Here's how the part is built. I have some questions about the finished solid (model axes, mm). Face numbers are marked on the shaded views. A direction names the side the tool comes from. Round coordinates to 2 decimals unless told otherwise and drop trailing zeros. Loops run counter-clockwise (first coordinate to the right, second up) from the corner with the lowest first, then second, coordinate; pieces in that order, holes last. Notation, with made-up numbers: (-12.5, -20) -> (15.5, -20) arc R22 ccw to (15.5, 14) -> close; hole circle Ø11 at (17.5, 25.5). An arc over 180 degrees is marked (long way). Use CSV: the item, a comma, the result in double quotes. Start each with the question number.
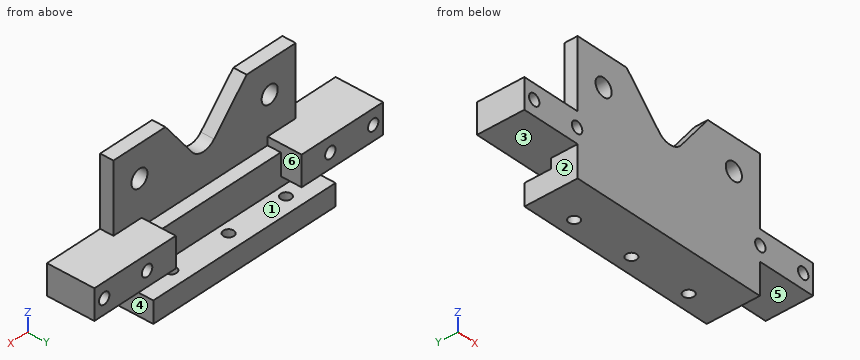
Autodesk Inventor part; units mm, degrees
ref_plane "YZ Plane" through (0, 0, 0) normal (1, 0, 0) x (0, 1, 0)
ref_plane "XZ Plane" through (0, 0, 0) normal (0, 1, 0) x (-1, 0, 0)
ref_plane "XY Plane" through (0, 0, 0) normal (0, 0, 1) x (1, 0, 0)
ref_plane "Work Plane1" through (-0.2015, 0, 0) normal (0, 0, 1) x (1, 0, 0)
sketch "Sketch1" plane through (-0.2015, 0, 0) normal (0, 0, 1) x (1, 0, 0)
  circle A0 centre (19.4801, 3.175) radius 1.0541
  circle A1 centre (44.8801, 3.175) radius 1.0541
  circle A2 centre (57.5801, 3.175) radius 1.0541 construction
  circle A3 centre (6.7801, 3.175) radius 1.0541 construction
  circle A4 centre (32.1801, 3.175) radius 1.0541
  line L0 (0.2015, 0) -> (64.1587, 0) construction
  line L1 (64.1587, 0) -> (64.1587, 6.35) construction
  line L2 (0.2015, 6.35) -> (64.1587, 6.35) construction
  line L3 (0.2015, 0) -> (0.2015, 6.35) construction
  line L4 (52.3672, 6.35) -> (11.9931, 6.35)
  line L5 (11.9931, 6.35) -> (11.9931, 0)
  line L6 (11.9931, 0) -> (52.3672, 0)
  line L7 (52.3672, 0) -> (52.3672, 6.35)
  line L8 (44.8801, 3.175) -> (52.3672, 3.175) construction
  line L9 (19.4801, 3.175) -> (11.9931, 3.175) construction
extrude "Extrusion1" add sketch "Sketch1" along normal blind 4.318
sketch "Sketch2" plane through (11.7916, 0, 0) normal (0, -1, 0) x (1, 0, 0)
  line L0 (0, 0) -> (40.3741, 0)
  line L1 (40.3741, 0) -> (40.3741, 4.318)
  line L2 (0, 4.318) -> (40.3741, 4.318)
  line L3 (0, 0) -> (0, 4.318)
  point P0 (-11.7916, 0)
extrude "Extrusion2" add sketch "Sketch2" along normal blind 4.318
sketch "Sketch3" plane through (-0.2015, 0, 4.318) normal (0, 0, 1) x (1, 0, 0)
  line L0 (52.3672, 6.35) -> (52.3672, -4.318)
  line L1 (52.3672, 1.016) -> (11.9931, 1.016)
  line L2 (11.9931, 6.35) -> (11.9931, -4.318)
  line L3 (52.3672, -4.318) -> (11.9931, -4.318)
  line L4 (52.3672, 1.016) -> (11.9931, 1.016)
  line L5 (11.9931, 1.016) -> (11.9931, -4.318)
  line L6 (11.9931, -4.318) -> (52.3672, -4.318)
  line L7 (52.3672, -4.318) -> (52.3672, 1.016)
  point P0 (0.2015, 0)
extrude "Extrusion3" add sketch "Sketch3" along normal blind 21.7805
sketch "Sketch4" plane through (11.7916, -4.318, 0) normal (0, -1, 0) x (1, 0, 0)
  line L0 (0, 0) -> (40.3741, 0) construction
  line L1 (40.3741, 0) -> (40.3741, 26.0985) construction
  line L2 (0, 26.0985) -> (40.3741, 26.0985) construction
  line L3 (0, 0) -> (0, 26.0985) construction
  line L4 (0, 26.0985) -> (40.3741, 26.0985) construction
  line L5 (28.8565, 26.0985) -> (22.9541, 18.3371)
  line L6 (18.0716, 18.1299) -> (10.868, 26.0985)
  line L7 (25.9053, 22.2178) -> (20.1871, 22.2178) construction
  line L8 (20.1871, 22.2178) -> (20.1871, 26.0985) construction
  line L9 (20.1871, 22.2178) -> (14.4698, 22.1142) construction
  line L10 (10.868, 26.0985) -> (28.8565, 26.0985)
  arc A0 (18.0716, 18.1299) -> (22.9541, 18.3371) centre (20.4268, 20.259) ccw
  point P0 (-11.7916, 0)
  point P1 (20.6377, 15.2912)
  dimension "d8" = 3.175
extrude "Extrusion4" cut sketch "Sketch4" against normal through all
sketch "Sketch5" plane through (11.7916, -4.318, 0) normal (0, -1, 0) x (1, 0, 0)
  line L0 (28.8565, 26.0985) -> (22.9541, 18.3371)
  arc A0 (18.0716, 18.1299) -> (22.9541, 18.3371) centre (20.4268, 20.259) ccw
  line L1 (18.0716, 18.1299) -> (10.868, 26.0985)
  line L2 (0, 26.0985) -> (10.868, 26.0985)
  line L3 (0, 0) -> (0, 26.0985)
  line L4 (0, 0) -> (40.3741, 0)
  line L5 (40.3741, 0) -> (40.3741, 26.0985)
  line L6 (28.8565, 26.0985) -> (40.3741, 26.0985)
  line L7 (40.3741, 0) -> (40.3741, 26.0985) construction
  line L8 (0, 4.318) -> (0, 26.0985) construction
  line L9 (40.3741, 19.7485) -> (0, 19.7485) construction
  line L10 (5.7588, 24.0238) -> (5.7588, 16.2202) construction
  line L11 (28.8565, 26.0985) -> (40.3741, 26.0985) construction
  line L12 (34.6153, 26.0985) -> (34.6153, 15.2083) construction
  line L13 (34.6153, 22.1235) -> (40.3741, 22.1235) construction
  line L14 (40.3741, 4.318) -> (40.3741, 26.0985) construction
  line L15 (5.7588, 22.1235) -> (0, 22.1235) construction
  line L16 (0, 0) -> (0, 26.0985) construction
  circle A1 centre (34.6153, 19.7485) radius 1.7859
  circle A2 centre (5.7588, 19.7485) radius 1.7859
  point P0 (-11.7916, 0)
  dimension "d10" = 6.35
  dimension "d16" = 3.5719
extrude "Extrusion5" cut sketch "Sketch5" against normal through all contours A1 | A2
sketch "Sketch6" plane through (-0.2015, 0, 26.0985) normal (0, 0, 1) x (1, 0, 0)
  line L0 (11.9931, 1.016) -> (11.9931, -4.318) construction
  line L1 (52.3672, -4.318) -> (52.3672, 1.016) construction
  circle A0 centre (32.1801, 3.175) radius 1.0541 construction
  circle A1 centre (44.8801, 3.175) radius 1.0541 construction
  circle A2 centre (19.4801, 3.175) radius 1.0541 construction
  line L2 (52.3672, 6.35) -> (11.9931, 6.35) construction
  line L3 (52.3672, 6.35) -> (52.3672, -4.318) construction
  line L4 (11.9931, -4.318) -> (52.3672, -4.318) construction
  line L5 (11.9931, 6.35) -> (11.9931, -4.318) construction
  line L6 (52.3672, -1.651) -> (11.9931, -1.651)
  line L7 (52.3672, -1.651) -> (11.9931, -1.651)
  line L8 (11.9931, -1.651) -> (11.9931, 6.35)
  line L9 (11.9931, 6.35) -> (52.3672, 6.35)
  line L10 (52.3672, 6.35) -> (52.3672, -1.651)
  point P0 (0.2015, 0)
extrude "Extrusion6" cut sketch "Sketch6" against normal blind 15.4305
sketch "Sketch7" plane through (11.7916, -4.318, 0) normal (0, -1, 0) x (1, 0, 0)
  line L0 (-11.7916, 6.2906) -> (6.2413, 6.2906)
  line L1 (6.2413, 6.2906) -> (6.2413, 12.2882)
  line L2 (6.2413, 12.2882) -> (-11.7916, 12.2882)
  line L3 (-11.7916, 12.2882) -> (-11.7916, 6.2906)
  point P0 (-11.7916, 0)
extrude "Extrusion7" add sketch "Sketch7" against normal blind 9.525
ref_plane "Work Plane2" through (31.9786, 3.175, 4.318) normal (1, 0, 0) x (0, 0, -1)
sketch "Sketch12" plane through (11.7916, -4.318, 0) normal (0, -1, 0) x (1, 0, 0)
  point P0 (-11.7916, 0)
mirror "Mirror2" about plane through (31.9786, 3.175, 4.318) normal (1, 0, 0) of "Extrusion7"
sketch "Sketch13" plane through (11.7916, -4.318, 0) normal (0, -1, 0) x (1, 0, 0)
  line L0 (40.3741, 12.2882) -> (40.3741, 26.0985) construction
  line L1 (28.8565, 26.0985) -> (40.3741, 26.0985) construction
  line L2 (28.8565, 26.0985) -> (22.9541, 18.3371) construction
  arc A0 (18.0716, 18.1299) -> (22.9541, 18.3371) centre (20.4268, 20.259) ccw construction
  line L3 (18.0716, 18.1299) -> (10.868, 26.0985) construction
  line L4 (0, 26.0985) -> (10.868, 26.0985) construction
  line L5 (0, 12.2882) -> (0, 26.0985) construction
  line L6 (0, 12.2882) -> (-11.7916, 12.2882) construction
  line L7 (-11.7916, 12.2882) -> (-11.7916, 6.2906) construction
  line L8 (-11.7916, 6.2906) -> (0, 6.2906) construction
  line L9 (0, 0) -> (0, 6.2906) construction
  line L10 (0, 0) -> (40.3741, 0) construction
  line L11 (40.3741, 0) -> (40.3741, 6.2906) construction
  line L12 (52.1657, 6.2906) -> (40.3741, 6.2906) construction
  line L13 (52.1657, 12.2882) -> (52.1657, 6.2906) construction
  line L14 (40.3741, 12.2882) -> (52.1657, 12.2882) construction
  circle A1 centre (5.7588, 19.7485) radius 1.7859 construction
  circle A2 centre (34.6153, 19.7485) radius 1.7859 construction
  line L15 (-11.7916, 9.2894) -> (52.1657, 9.2894) construction
  circle A3 centre (-9.6132, 9.2894) radius 1.15
  circle A4 centre (-0.1136, 9.2894) radius 1.15
  line L16 (-9.6132, 9.2894) -> (-9.6132, 7.1957) construction
  line L17 (-0.1136, 9.2894) -> (-0.1136, 7.1957) construction
  point P0 (-11.7916, 0)
  dimension "d22" = 9.4996
  dimension "d23" = 2.3
extrude "Extrusion9" cut sketch "Sketch13" against normal through all
mirror "Mirror3" about plane through (31.9786, 3.175, 4.318) normal (1, 0, 0) of "Extrusion9"
properties part number "bumper lever support"
Q1. For the marked faces 1, 2 and 3, which set-ups out of +Z, -Z, +X, -X, +Y, -Y let a thin tool reach every point of the face, with its end or its side?
Q2. If we mould it in two halves opening along X, with no side actions, what happens to the marked faces 4, 5 and 6? For each: pulls with the +X half, pulls with the -X half, needs draft (parallel to the pull), parting line crosses it, or undercut.
Q3. I want a section at C-C, the plane x = 49. List the corners of the cut face in (y, z) for me.
Q4. Will these pins go through, and if not, where does the flat tip stop? pin 1 Ø5 at (y, z) = (1, 3) entering from +X; pin 2 Ø1 at (x, y) = (36, 0.5) entering from +Z; pin 3 Ø3 at (y, z) = (0, 14) entering from -X; pin 4 Ø3 at (x, z) = (11.68, 9.29) entering from +Y.
Q5. I want a section at D-D, the plane y = 0. List the corners of the cut face in (x, z) for me.
Q6. I want a section at B-B, the plane z = 24.25. List the corners of the cut face in (x, y) for me.
Q7. I need wall thicknesses on line 1 along Z through (x, y) = (42, 4.5); line 2 along Z through (x, y) = (17.5, 0.25); line 3 along X through (y, z) = (-3.5, 19.25). Which ranges of each line are inside material? Lowest first, please.
Q8. I want a section at A-A, the plane x = 17. List the corners of the cut face in (y, z) for me, then the cut area to 3 significant figures.
Values found:
1,face 1,"+X, -X, +Y"
1,face 2,"-Z, -X, +Y, -Y"
1,face 3,"-X, +Y"
2,face 4,"pulls with the +X half"
2,face 5,"needs draft"
2,face 6,"undercut"
3,outline,"(-4.32, 0) -> (6.35, 0) -> (6.35, 4.32) -> (1.02, 4.32) -> (1.02, 6.29) -> (5.21, 6.29) -> (5.21, 12.29) -> (-1.65, 12.29) -> (-1.65, 26.1) -> (-4.32, 26.1) -> close"
4,pin 1,"x = 52.17"
4,pin 2,"z = 10.67"
4,pin 3,"through"
4,pin 4,"y = 5.21"
5,outline,"(0, 6.29) -> (11.79, 6.29) -> (11.79, 0) -> (52.17, 0) -> (52.17, 6.29) -> (63.96, 6.29) -> (63.96, 12.29) -> (45.92, 12.29) -> (45.92, 10.67) -> (18.03, 10.67) -> (18.03, 12.29) -> (0, 12.29) -> close; hole circle Ø2.3 at (2.18, 9.29); hole circle Ø2.3 at (11.68, 9.29); hole circle Ø2.3 at (52.28, 9.29); hole circle Ø2.3 at (61.78, 9.29)"
6,outline,"(11.79, -4.32) -> (24.33, -4.32) -> (24.33, -1.65) -> (11.79, -1.65) -> close; (39.24, -4.32) -> (52.17, -4.32) -> (52.17, -1.65) -> (39.24, -1.65) -> close"
7,line 1,"0 to 4.32"
7,line 2,"0 to 12.29"
7,line 3,"11.79 to 15.84, 19.27 to 28.85, 35.44 to 44.69, 48.12 to 52.17"
8,outline,"(-4.32, 0) -> (6.35, 0) -> (6.35, 4.32) -> (1.02, 4.32) -> (1.02, 6.29) -> (5.21, 6.29) -> (5.21, 12.29) -> (-1.65, 12.29) -> (-1.65, 18.05) -> (-4.32, 18.05) -> close; (-4.32, 21.45) -> (-1.65, 21.45) -> (-1.65, 26.1) -> (-4.32, 26.1) -> close"
8,area,"141 mm2"
